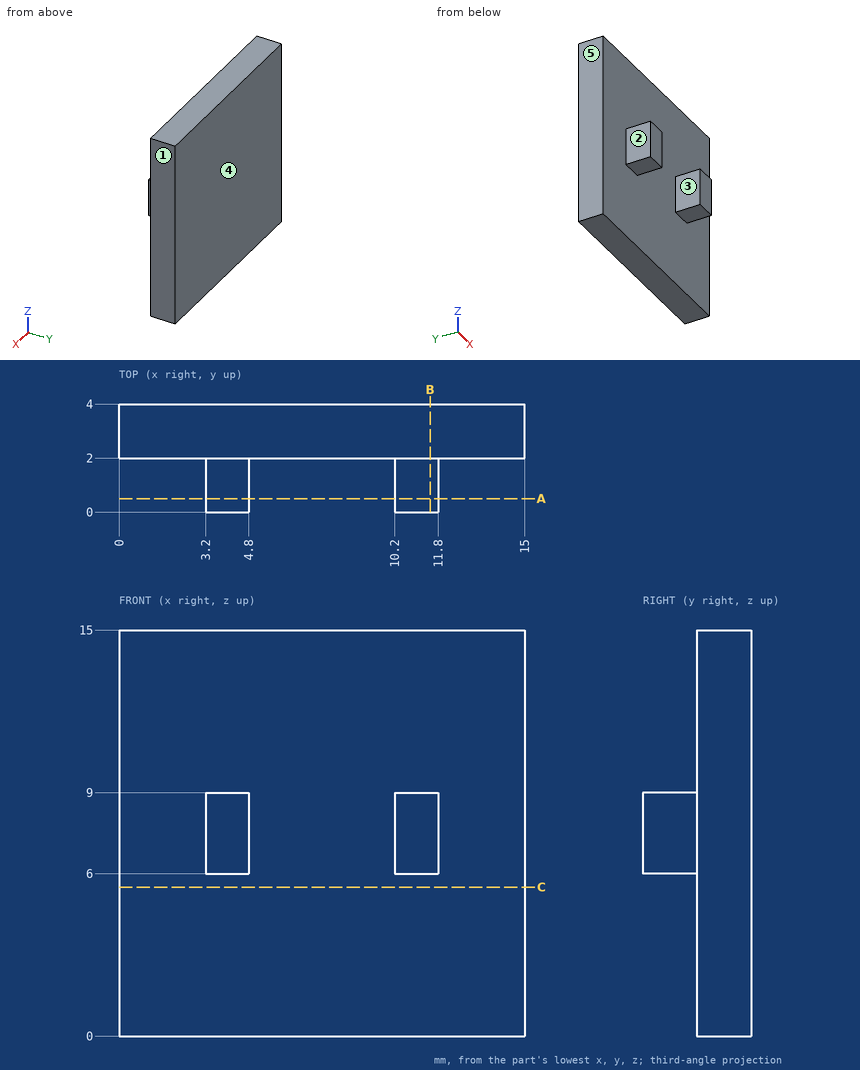
Design review of the part shown in the three views and the two pictorial views. Dimensions are in mm from the part's minimum x, y and z. A direction names the side the tool comes from. Coordinates: 2 decimals unless noted, no trailing zeros. Write each loop counter-clockwise with the first axis right and the second up, starting at its lowest first coordinate (ties: lowest second). Pieces come first, ordered by that corner, then holes.
1) The part is to be moulded in two halves that separate along X. For the marked faces 3, 4 and 5, say which applies: pulls with the +X half, pulls with the -X half, needs draft (parallel to the pull), parting line crosses it, or undercut.
2) Clearance check with flat-ended pins moving along their axes: pin 1 Ø1.3 at (x, y) = (11, 1) entering from -Z; pin 2 Ø1 at (y, z) = (1, 8) entering from +X; pin 3 Ø0.5 at (x, y) = (10.5, 1) entering from +Z. State where each tip first meets the part, or that it passes through.
3) We need section B-B on x = 11.5. State the section outline as (y, z) points, then the cut area to 3 significant figures.
4) Machinability: for the marked faces 1 and 2, which of the approach directions +Z, -Z, +X, -X, +Y, -Y give a long, thin tool a straight path to every point of the face, cutting with its end or side? Answer none if there is none.
5) We need section C-C on z = 5.5. State the section outline as (x, y) points, then the cut area to 3 significant figures.
6) We need section A-A on y = 0.5. State the section outline as (x, z) points, then the cut area to 3 significant figures.
7) To check wall thickness, follow probe 1 along X at (y, z) = (0.4, 8); probe 2 along Y at (x, z) = (9.25, 3.5); probe 3 along Z at (x, y) = (10.5, 1.05). State the ranges of each line that lie inside material, in increasing order.
Answer list:
1. face 3: undercut
1. face 4: needs draft
1. face 5: pulls with the -X half
2. pin 1: stops at z = 6
2. pin 2: stops at x = 11.8
2. pin 3: stops at z = 9
3. outline: (0, 6) - (2, 6) - (2, 0) - (4, 0) - (4, 15) - (2, 15) - (2, 9) - (0, 9) - close
3. area: 36.0 mm2
4. face 1: +Z, -Z, +X, +Y, -Y
4. face 2: +Z, -Z, -X, -Y
5. outline: (0, 2) - (15, 2) - (15, 4) - (0, 4) - close
5. area: 30.0 mm2
6. outline: (3.2, 6) - (4.8, 6) - (4.8, 9) - (3.2, 9) - close; (10.2, 6) - (11.8, 6) - (11.8, 9) - (10.2, 9) - close
6. area: 9.60 mm2
7. probe 1: x = 3.2 to 4.8, 10.2 to 11.8
7. probe 2: y = 2 to 4
7. probe 3: z = 6 to 9
